CAD build for the part. Positions are in the model's coordinates, mm. A direction names the side the tool comes from. Round coordinates to 2 decimals unless told otherwise and drop trailing zeros. Write each loop counter-clockwise with the first axis right and the second up, starting at its lowest first coordinate (ties: lowest second). Pieces come first, ordered by that corner, then holes. Notation, with made-up numbers: (-10, -22.5) -> (11, -22.5) arc R28 cw to (11, 1.5) -> close; hole circle Ø1 at (34.5, 78). An arc over 180 degrees is marked (long way). Put each result on its own line as item: value. Start each with the question number.
1. Saw through at A-A on z = -35. List the corners of the cut face in (x, y), and give its area (3 significant figures).
2. Saw through at B-B on x = 37.5. List the corners of the cut face in (y, z).
3. Pull direction Z, two halves, no side cores. Call faces 1 (the cylindrical face through (68.986, 3.131, -69.297)), 2 (the flat face through (-75, 3, 1)), 3 (the cylindrical face through (-68.986, 3.131, 69.297)), 4 (the flat face through (34.5, 3, 37)): pulls with the +Z half, pulls with the -Z half, needs draft (parallel to the pull), parting line crosses it, or undercut.
4. Saw through at C-C on y = 2.25. State how many separate pieces and enclosed holes the cut face has, and give its area (3 significant figures).
5. Saw through at D-D on z = -63. List the corners of the cut face in (x, y), and give its area (3 significant figures).
6. 3-axis set-ups, long thin cutter, end or side, ignore diameter. For faces 5 (the cylindrical face through (-37.6, 3.2, 45.5)), 6 (the flat face through (-1, 3, -75)): which of +Z, -Z, +X, -X, +Y, -Y reach the whole face in a straight line?
7. Drill centre lines: line 1 (X direction, y = 4.5, z = 50); line 2 (X direction, y = 3, z = 38.5). Where is each one in solid material? Low to high. Write a range as from..to.
from build123d import *

# Parameters (mm, degrees)
SKETCH1_R           = 1.5
BOSS_EXTRUDE1_DEPTH = 6.35
CUT_EXTRUDE1_DEPTH  = 10


with BuildPart() as part:
    # Sketch1 → Boss-Extrude1 (new body)
    with BuildSketch(Plane(origin=(0, 0, 0), x_dir=(1, 0, 0), z_dir=(0, 1, 0))):
        with BuildLine():
            Line((-55, 75), (55, 75))
            ThreePointArc((55, 75), (69.142135624, 69.142135624), (75, 55))
            Line((75, 55), (75, -55))
            ThreePointArc((75, -55), (69.142135624, -69.142135624), (55, -75))
            Line((55, -75), (-55, -75))
            ThreePointArc((-55, -75), (-69.142135624, -69.142135624), (-75, -55))
            Line((-75, -55), (-75, 55))
            ThreePointArc((-75, 55), (-69.142135624, 69.142135624), (-55, 75))
        make_face()
        with Locations((50, 50)):
            Circle(SKETCH1_R, mode=Mode.SUBTRACT)
        with Locations((50, -50)):
            Circle(SKETCH1_R, mode=Mode.SUBTRACT)
        with Locations((-50, -50)):
            Circle(SKETCH1_R, mode=Mode.SUBTRACT)
        with Locations((-50, 50)):
            Circle(SKETCH1_R, mode=Mode.SUBTRACT)
    extrude(amount=BOSS_EXTRUDE1_DEPTH)

    # Sketch2 → Cut-Extrude1 (cut)
    with BuildSketch(Plane(origin=(0, 6.35, 0), x_dir=(1, 0, 0), z_dir=(0, 1, 0))):
        with BuildLine():
            Line((40.5, 42.5), (40.5, 32.5))
            ThreePointArc((40.5, 32.5), (37.5, 29.5), (34.5, 32.5))
            Line((34.5, 32.5), (34.5, 42.5))
            ThreePointArc((34.5, 42.5), (37.5, 45.5), (40.5, 42.5))
        make_face()
        with BuildLine():
            Line((-34.5, 42.5), (-34.5, 32.5))
            ThreePointArc((-34.5, 32.5), (-37.5, 29.5), (-40.5, 32.5))
            Line((-40.5, 32.5), (-40.5, 42.5))
            ThreePointArc((-40.5, 42.5), (-37.5, 45.5), (-34.5, 42.5))
        make_face()
        with BuildLine():
            Line((40.5, -42.5), (40.5, -32.5))
            ThreePointArc((40.5, -32.5), (37.5, -29.5), (34.5, -32.5))
            Line((34.5, -32.5), (34.5, -42.5))
            ThreePointArc((34.5, -42.5), (37.5, -45.5), (40.5, -42.5))
        make_face()
        with BuildLine():
            Line((-34.5, -42.5), (-34.5, -32.5))
            ThreePointArc((-34.5, -32.5), (-37.5, -29.5), (-40.5, -32.5))
            Line((-40.5, -32.5), (-40.5, -42.5))
            ThreePointArc((-40.5, -42.5), (-37.5, -45.5), (-34.5, -42.5))
        make_face()
    extrude(amount=-CUT_EXTRUDE1_DEPTH, mode=Mode.SUBTRACT)


solid = part.part
Return value:
1. outline: (-75, 0) -> (-40.5, 0) -> (-40.5, 6.35) -> (-75, 6.35) -> close; (-34.5, 0) -> (34.5, 0) -> (34.5, 6.35) -> (-34.5, 6.35) -> close; (40.5, 0) -> (75, 0) -> (75, 6.35) -> (40.5, 6.35) -> close
1. area: 876 mm^2
2. outline: (0, -75) -> (6.35, -75) -> (6.35, -45.5) -> (0, -45.5) -> close; (0, -29.5) -> (6.35, -29.5) -> (6.35, 29.5) -> (0, 29.5) -> close; (0, 45.5) -> (6.35, 45.5) -> (6.35, 75) -> (0, 75) -> close
3. face 1: pulls with the -Z half
3. face 2: needs draft
3. face 3: pulls with the +Z half
3. face 4: undercut
4. separate pieces: 1
4. enclosed holes: 8
4. area: 21,800 mm^2
5. outline: (-73.33, 0) -> (73.33, 0) -> (73.33, 6.35) -> (-73.33, 6.35) -> close
5. area: 931 mm^2
6. face 5: +Y, -Y
6. face 6: -Z, +X, -X, +Y, -Y
7. line 1: x = -75..-51.5, -48.5..48.5, 51.5..75
7. line 2: x = -75..-40.5, -34.5..34.5, 40.5..75
